from build123d import *

# Parameters (mm, degrees)
SKETCH2_W  = 19.05
SKETCH2_H  = 2.6924
SLOT_DEPTH = 4.826


with BuildPart() as part:
    # BodySke → Base-Revolve (revolve)
    with BuildSketch(Plane.XY, mode=Mode.PRIVATE) as base_revolve_sk:
        with BuildLine():
            Line((10.4648, 6.35), (10.4648, 9.525))
            Line((10.4648, 9.525), (2.921, 9.525))
            ThreePointArc((2.921, 9.525), (0.746656199, 4.981412099), (0, 0))
            Line((0, 0), (61.2648, 0))
            Line((61.2648, 0), (61.2648, 6.35))
            Line((61.2648, 6.35), (10.4648, 6.35))
        make_face()
    revolve(base_revolve_sk.sketch.rotate(Axis((-25.4, 0, 0), (1, 0, 0)), 90), axis=Axis((-25.4, 0, 0), (1, 0, 0)))

    # Sketch2 → Slot (cut)
    with BuildSketch(Plane(origin=(0, 0, 0), x_dir=(0, 0, -1), z_dir=(1, 0, 0))):
        Rectangle(SKETCH2_W, SKETCH2_H)
    extrude(amount=SLOT_DEPTH, mode=Mode.SUBTRACT)


solid = part.part
Model file for the job. Use its own axes, mm. A direction names the side the tool comes from. Round coordinates to 2 decimals unless told otherwise and drop trailing zeros. Order: outer loops, then holes, each group sorted by start corner. A loop starts at its lowest first (then second) coordinate and runs counter-clockwise, first axis right, second up.
(1) Band-saw the part on D-D (z = -8.5). List the corners of the cut face in (x, y), then the cut area to 3 significant figures.
(2) Pin check, flat tips, straight feed: pin 1 (10 mm diameter, centred on x = 23, z = -2.5, fed in from +Y); pin 2 (0.8 mm diameter, centred on y = 0.5, z = -0.5, fed in from -X); pin 3 (5 mm diameter, centred on x = 1.5, z = 3.5, fed in from -Y). Stop position of each tip, or through.
(3) Drill centre lines: line 1 (X direction, y = -0.75, z = 3.75); line 2 (Z direction, x = 26, y = -0.25); line 3 (Y direction, x = 3, z = -7.75). Where is each one in solid material? Low to high.
(4) Band-saw the part on C-C (x = 38). List the corners of the cut face in (y, z), then the cut area to 3 significant figures.
(5) Band-saw the part on B-B (z = 0). List the corners of the cut face in (x, y) (3 decimals), then the cut area to 3 significant figures.
(6) Band-saw the part on A-A (y = 0). List the corners of the cut face in (x, z) (3 decimals), then the cut area to 3 significant figures.
(7) 3-axis set-ups, long thin cutter, end or side, ignore diameter. For faces 4 (the face through (6.64, -2.861, 9.085)), 5 (the face through (10.465, 2, -6.2)), 6 (the face through (4.826, 0, 0)): which of +Z, -Z, +X, -X, +Y, -Y reach the whole face in a straight line?
(8) Pull direction Y, two halves, no side cores. Call faces 1 (the face through (61.265, 0, 0)), 2 (the face through (35.51, 3.86, -5.04)), 3 (the face through (3, -1.346, 0)): released by +Y, released by -Y, zero draft, split by the parting line, or undercut.
Verdict:
1. outline: (2.34, -1.35) arc R14.71 ccw to (2.92, -4.3) - (10.46, -4.3) - (10.46, 4.3) - (2.92, 4.3) arc R14.71 ccw to (2.34, 1.35) - (4.83, 1.35) - (4.83, -1.35) - close
1. area: 61.7 mm2
2. pin 1: stops at y = 6.35
2. pin 2: stops at x = 4.83
2. pin 3: stops at y = -9.42
3. line 1: x = 4.83 to 61.26
3. line 2: z = -6.35 to 6.35
3. line 3: y = -5.54 to -1.35, 1.35 to 5.54
4. outline: circle Ø12.7 at (0, 0)
4. area: 127 mm2
5. outline: (0.053, -1.346) arc R16.99 ccw to (2.921, -9.525) - (10.465, -9.525) - (10.465, -6.35) - (61.265, -6.35) - (61.265, 6.35) - (10.465, 6.35) - (10.465, 9.525) - (2.921, 9.525) arc R16.99 ccw to (0.053, 1.346) - (4.826, 1.346) - (4.826, -1.346) - close
5. area: 814 mm2
6. outline: (4.826, -9.525) - (10.465, -9.525) - (10.465, -6.35) - (61.265, -6.35) - (61.265, 6.35) - (10.465, 6.35) - (10.465, 9.525) - (4.826, 9.525) - close
6. area: 753 mm2
7. face 4: +X, -X
7. face 5: +X
7. face 6: +Z, -Z, -X
8. face 1: zero draft
8. face 2: split by the parting line
8. face 3: undercut
